Build history of the part. All positions in model axes, mm. Face numbers are marked on the shaded views. A direction names the side the tool comes from. Give positions to 0.01 mm unless a question says otherwise; leave off trailing zeros. Write each loop counter-clockwise with the first axis right and the second up, starting at its lowest first coordinate (ties: lowest second). Pieces come first, ordered by that corner, then holes. Notation, with made-up numbers: M -4.5,19.25 L 1.5,19.25 A29 cw 1.5,51.25 Z; hole C 2.25,35 d1. An arc over 180 degrees is marked long. Return JSON: item names as keys, results as strings. Group by question number.
Q1. Band-saw the part on C-C, the plane z = 36. Give the cut face in (x, y), then the cut area to 3 significant figures.
Q2. Wall check: probe 1 along X at (y, z) = (161.2, 74.5); probe 2 along Z at (x, y) = (-97, 161); probe 3 along Z at (x, y) = (-92, 87.5). Give the ranges that are in metal, low to high.
Q3. Flat gauge pins, fed straight in: pin 1 Ø12 at (y, z) = (-21, 21) entering from +X; pin 2 Ø13.5 at (x, y) = (1, 105.5) entering from -Z; pin 3 Ø1 at (y, z) = (161, 17.5) entering from +X; pin 4 Ø4 at (x, y) = (90.97, -52.43) entering from -Z. Where does each tip first touch, or does it go through?
Q4. Tool access for the marked faces 4, 5, 6 and 7: list every direction of +Z, -Z, +X, -X, +Y, -Y with a clear straight run to the whole face (end or side of a thin tool).
Q5. Pull direction X, two halves, no side cores. Call the marked faces 1, 2 and 3: +X half, -X half, draft (parallel to the pull), parting line (faces both ways), or undercut.
Q6. Band-saw the part on A-A, the plane y = 129.5. Give the cut face in (x, z), then the cut area to 3 significant figures.
Q7. Band-saw the part on B-B, the plane x = 60. Give the cut face in (y, z), then the cut area to 3 significant figures.
Q8. Band-saw the part on D-D, the plane y = -15. Give the cut face in (x, z), then the cut area to 3 significant figures.
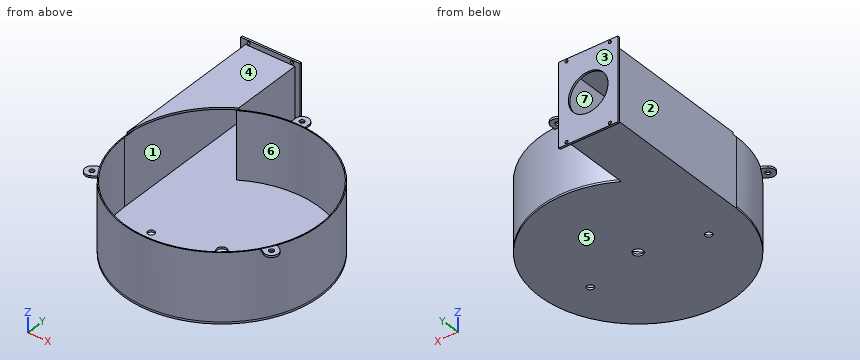
from build123d import *

# Parameters (mm, degrees)
IZIM1_R                     = 3.5
IZIM1_R_2                   = 5
Y_KSEKLIK_EKSTR_ZYON1_DEPTH = 2
Y_KSEKLIK_EKSTR_ZYON3_DEPTH = 68
Y_KSEKLIK_EKSTR_ZYON4_DEPTH = 2
Y_KSEKLIK_EKSTR_ZYON6_START = -2
IZIM6_R                     = 2.5
Y_KSEKLIK_EKSTR_ZYON6_DEPTH = 2
IZIM8_W                     = 60
IZIM8_H                     = 84
IZIM8_R                     = 20.122069198
IZIM8_R_2                   = 1.5
Y_KSEKLIK_EKSTR_ZYON7_DEPTH = 2


with BuildPart() as part:
    # Çizim1 → Yükseklik-Ekstrüzyon1 (new body)
    with BuildSketch(Plane.XY):
        with BuildLine():
            Line((-100, 0), (-100, 160))
            Line((-100, 160), (-50, 160))
            Line((-50, 160), (-50, 86.602540378))
            ThreePointArc((-50, 86.602540378), (86.602540378, -50), (-100, 0))
        make_face()
        with Locations((-60, -15)):
            Circle(IZIM1_R, mode=Mode.SUBTRACT)
        with Locations((60, -15)):
            Circle(IZIM1_R, mode=Mode.SUBTRACT)
        Circle(IZIM1_R_2, mode=Mode.SUBTRACT)
    extrude(amount=Y_KSEKLIK_EKSTR_ZYON1_DEPTH)

    # Çizim2 → Yükseklik-Ekstrüzyon3 (add)
    with BuildSketch(Plane.XY.offset(2)):
        with BuildLine():
            Line((-50, 86.602540378), (-50, 160))
            Line((-50, 160), (-51, 160))
            Line((-51, 160), (-51, 159))
            Line((-51, 159), (-51, 84.852813742))
            ThreePointArc((-51, 84.852813742), (86.168439698, -48.744230428), (-99, 0))
            Line((-99, 0), (-99, 159))
            Line((-99, 159), (-99, 160))
            Line((-99, 160), (-100, 160))
            Line((-100, 160), (-100, 0))
            ThreePointArc((-100, 0), (86.602540378, -50), (-50, 86.602540378))
        make_face()
    extrude(amount=Y_KSEKLIK_EKSTR_ZYON3_DEPTH)

    # Çizim4 → Yükseklik-Ekstrüzyon4 (add)
    with BuildSketch(Plane.XY.offset(70)):
        with BuildLine():
            Line((-100, 160), (-50, 160))
            Line((-50, 160), (-50, 86.602540378))
            ThreePointArc((-50, 86.602540378), (-85.384878706, 52.052113198), (-99.88613884, 4.77066743))
            Line((-99.88613884, 4.77066743), (-100, 4.77066743))
            Line((-100, 4.77066743), (-100, 160))
        make_face()
    extrude(amount=Y_KSEKLIK_EKSTR_ZYON4_DEPTH)

    # Çizim6 → Yükseklik-Ekstrüzyon6 (add)
    # profile 1 of 3: a face of its own
    with BuildSketch(Plane.XY.offset(70).offset(Y_KSEKLIK_EKSTR_ZYON6_START)):
        with BuildLine():
            ThreePointArc((-7, 99.754699137), (-0.077865091, 99.999969685), (6.844643384, 99.765479285))
            Line((6.844643384, 99.765479285), (6.844643384, 106.039933839))
            ThreePointArc((6.844643384, 106.039933839), (-0.077678308, 112), (-7, 106.039933839))
            Line((-7, 106.039933839), (-7, 99.754699137))
        make_face()
        with Locations((-0.077678308, 105)):
            Circle(IZIM6_R, mode=Mode.SUBTRACT)
    # profile 2 of 3: a face of its own
    with BuildSketch(Plane.XY.offset(70).offset(Y_KSEKLIK_EKSTR_ZYON6_START)):
        with BuildLine():
            Line((-88.33327652, -59.082144746), (-82.8901036, -55.939527395))
            ThreePointArc((-82.8901036, -55.939527395), (-86.563581579, -50.067417989), (-89.821761174, -43.955104592))
            Line((-89.821761174, -43.955104592), (-95.255598212, -47.092331869))
            ThreePointArc((-95.255598212, -47.092331869), (-96.95600607, -56.067271388), (-88.33327652, -59.082144746))
        make_face()
        with Locations((-90.893828243, -52.567271388)):
            Circle(IZIM6_R, mode=Mode.SUBTRACT)
    # profile 3 of 3: a face of its own
    with BuildSketch(Plane.XY.offset(70).offset(Y_KSEKLIK_EKSTR_ZYON6_START)):
        with BuildLine():
            ThreePointArc((88.410954828, -58.94760197), (97.033684378, -55.932728612), (95.33327652, -46.957789093))
            Line((95.33327652, -46.957789093), (89.8901036, -43.815171742))
            ThreePointArc((89.8901036, -43.815171742), (86.641446671, -49.932551696), (82.977117789, -55.810374693))
            Line((82.977117789, -55.810374693), (88.410954828, -58.94760197))
        make_face()
        with Locations((90.971506551, -52.432728612)):
            Circle(IZIM6_R, mode=Mode.SUBTRACT)
    extrude(amount=Y_KSEKLIK_EKSTR_ZYON6_DEPTH)

    # Çizim8 → Yükseklik-Ekstrüzyon7 (add)
    with BuildSketch(Plane(origin=(0, 160, 0), x_dir=(1, 0, 0), z_dir=(0, 1, 0))):
        with Locations((-75, -35)):
            Rectangle(IZIM8_W, IZIM8_H)
        with Locations(Location((-75, -35, 0), (0, 0, 270))):
            Circle(IZIM8_R, mode=Mode.SUBTRACT)
        with Locations(Location((-97, 4.5, 0), (0, 0, 270))):
            Circle(IZIM8_R_2, mode=Mode.SUBTRACT)
        with Locations(Location((-53, 4.5, 0), (0, 0, 270))):
            Circle(IZIM8_R_2, mode=Mode.SUBTRACT)
        with Locations(Location((-53, -74.5, 0), (0, 0, 270))):
            Circle(IZIM8_R_2, mode=Mode.SUBTRACT)
        with Locations(Location((-97, -74.5, 0), (0, 0, 270))):
            Circle(IZIM8_R_2, mode=Mode.SUBTRACT)
    extrude(amount=Y_KSEKLIK_EKSTR_ZYON7_DEPTH)


solid = part.part
From the geometry:
{
 "1": {"outline": "M -105,160 L -100,160 L -100,0 A100 ccw long -50,86.6 L -50,160 L -45,160 L -45,162 L -54.9,162 L -54.9,160 L -51,160 L -51,84.85 A99 cw long -99,0 L -99,160 L -95.1,160 L -95.1,162 L -105,162 Z", "area": "796 mm^2"},
 "2": {"probe 1": "x = -105 to -98.5, -95.5 to -54.5, -51.5 to -45", "probe 2": "z = -7 to -6, -3 to 73, 76 to 77", "probe 3": "z = 0 to 2, 70 to 72"},
 "3": {"pin 1": "stops at x = 98.87", "pin 2": "stops at z = 0", "pin 3": "stops at x = -45", "pin 4": "passes through"},
 "4": {"face 4": "+Z, +X, -X, -Y", "face 5": "-Z, +X, -X, -Y", "face 6": "+Z", "face 7": "none"},
 "5": {"face 1": "undercut", "face 2": "-X half", "face 3": "draft"},
 "6": {"outline": "M -100,0 L -50,0 L -50,72 L -100,72 Z; hole M -99,2 L -51,2 L -51,70 L -99,70 Z", "area": "336 mm^2"},
 "7": {"outline": "M -80,0 L -18.5,0 L -18.5,2 L -78.75,2 L -78.75,70 L -80,70 Z; M -11.5,0 L 80,0 L 80,70 L 78.75,70 L 78.75,2 L -11.5,2 Z", "area": "476 mm^2"},
 "8": {"outline": "M -98.87,0 L -63.5,0 L -63.5,2 L -97.86,2 L -97.86,70 L -98.87,70 Z; M -56.5,0 L 56.5,0 L 56.5,2 L -56.5,2 Z; M 63.5,0 L 98.87,0 L 98.87,70 L 97.86,70 L 97.86,2 L 63.5,2 Z", "area": "505 mm^2"}
}
